Source: three-view drawing plus pictorial views. Frame: mm from the lowest corner of the part. Round coordinates to 2 decimals unless told otherwise and drop trailing zeros. Loops run counter-clockwise (first coordinate to the right, second up) from the corner with the lowest first, then second, coordinate; pieces in that order, holes last. Notation, with made-up numbers: (-30.75, 77.25) -> (-25.75, 77.25) arc R13 cw to (-25.75, 84.25) -> close; hole circle Ø9 at (-23, 32). An arc over 180 degrees is marked (long way). Put each result on its own line as item: value. Start each with the question number.
1. Cut plane C-C (z = 124). Return the cut outline in (x, y).
2. Material intervals for L1, parallel to Z at x = 144, y = 68.5; L2, parallel to X at y = 65.5, z = 22.5, sorted ascending.
3. Contact query for flat-ended pins moving along their axis: pin 1 (1.5 mm diameter, centred on x = 15.5, z = 81, fed in from -Y); pin 2 (1.6 mm diameter, centred on x = 149, z = 149.5, fed in from -Y). Output: stop coordinate, or through.
4. Cut plane B-B (x = 13). Return the cut outline in (y, z).
5. Cut plane D-D (z = 76.5). Return the cut outline in (x, y).
6. Cut plane A-A (y = 31). Return the cut outline in (x, z).
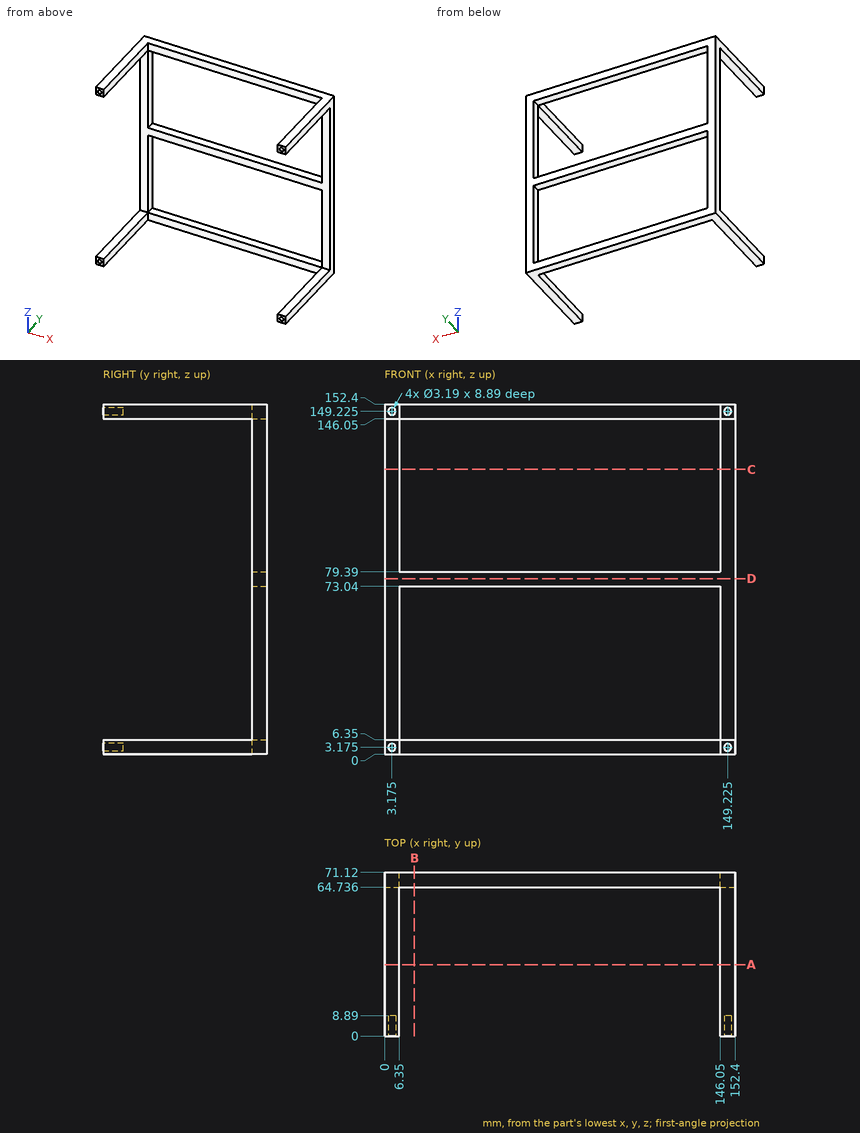
Solution:
1. outline: (0, 64.74) -> (6.35, 64.74) -> (6.35, 71.12) -> (0, 71.12) -> close; (146.05, 64.74) -> (152.4, 64.74) -> (152.4, 71.12) -> (146.05, 71.12) -> close
2. L1: z = 0 to 6.35, 73.04 to 79.39, 146.05 to 152.4
2. L2: x = 0 to 6.35, 146.05 to 152.4
3. pin 1: passes through
3. pin 2: stops at y = 8.89
4. outline: (64.74, 0) -> (71.12, 0) -> (71.12, 6.35) -> (64.74, 6.35) -> close; (64.74, 73.04) -> (71.12, 73.04) -> (71.12, 79.39) -> (64.74, 79.39) -> close; (64.74, 146.05) -> (71.12, 146.05) -> (71.12, 152.4) -> (64.74, 152.4) -> close
5. outline: (0, 64.74) -> (152.4, 64.74) -> (152.4, 71.12) -> (0, 71.12) -> close
6. outline: (0, 0) -> (6.35, 0) -> (6.35, 6.35) -> (0, 6.35) -> close; (0, 146.05) -> (6.35, 146.05) -> (6.35, 152.4) -> (0, 152.4) -> close; (146.05, 0) -> (152.4, 0) -> (152.4, 6.35) -> (146.05, 6.35) -> close; (146.05, 146.05) -> (152.4, 146.05) -> (152.4, 152.4) -> (146.05, 152.4) -> close
